Drawing for the job (mm, zero at the part's lowest x, y, z). A direction names the side the tool comes from. Give positions to 0.01 mm unless a question says otherwise; leave off trailing zeros. Write each loop counter-clockwise with the first axis right and the second up, starting at its lowest first coordinate (ties: lowest second). Pieces come first, ordered by that corner, then holes. Notation, with made-up numbers: M 1.25,-2.75 L 56.25,-2.75 A22 cw 56.25,24.25 Z; hole C 43.25,-3.5 d2. An arc over 180 degrees is marked long. Use CSV: the item, a comma, the result in double quotes. Start each with the question number.
1. Mould opens along X. For the marked faces 1, 2 and 3 say: pulls with the +X half, pulls with the -X half, needs draft (parallel to the pull), parting line crosses it, or undercut.
2. 3-axis set-ups, long thin cutter, end or side, ignore diameter. For the marked faces 4 and 5: which of +Z, -Z, +X, -X, +Y, -Y reach the whole face in a straight line?
3. Band-saw the part on A-A, the plane x = 12. List the corners of the cut face in (y, z).
4. Band-saw the part on C-C, the plane y = 0.5. List the corners of the cut face in (x, z), then the cut area to 3 significant figures.
5. Band-saw the part on D-D, the plane y = 8. List the corners of the cut face in (x, z).
6. Band-saw the part on B-B, the plane z = 12. List the corners of the cut face in (x, y), then the cut area to 3 significant figures.
7. Drop flat-ended pins along their axis: pin 1 Ø6 at (y, z) = (1, 17.5) entering from -X; pin 2 Ø8.5 at (x, z) = (12, 12) entering from -Y; pin 3 Ø1.5 at (y, z) = (9, 3) entering from -X. Give the stop position or say it passes through.
8. Drill centre lines: line 1 along Z through (x, y) = (12, 3.55); line 2 along Z through (x, y) = (12, 5.3). Where is each one in solid material? Low to high. Write a range as from..to.
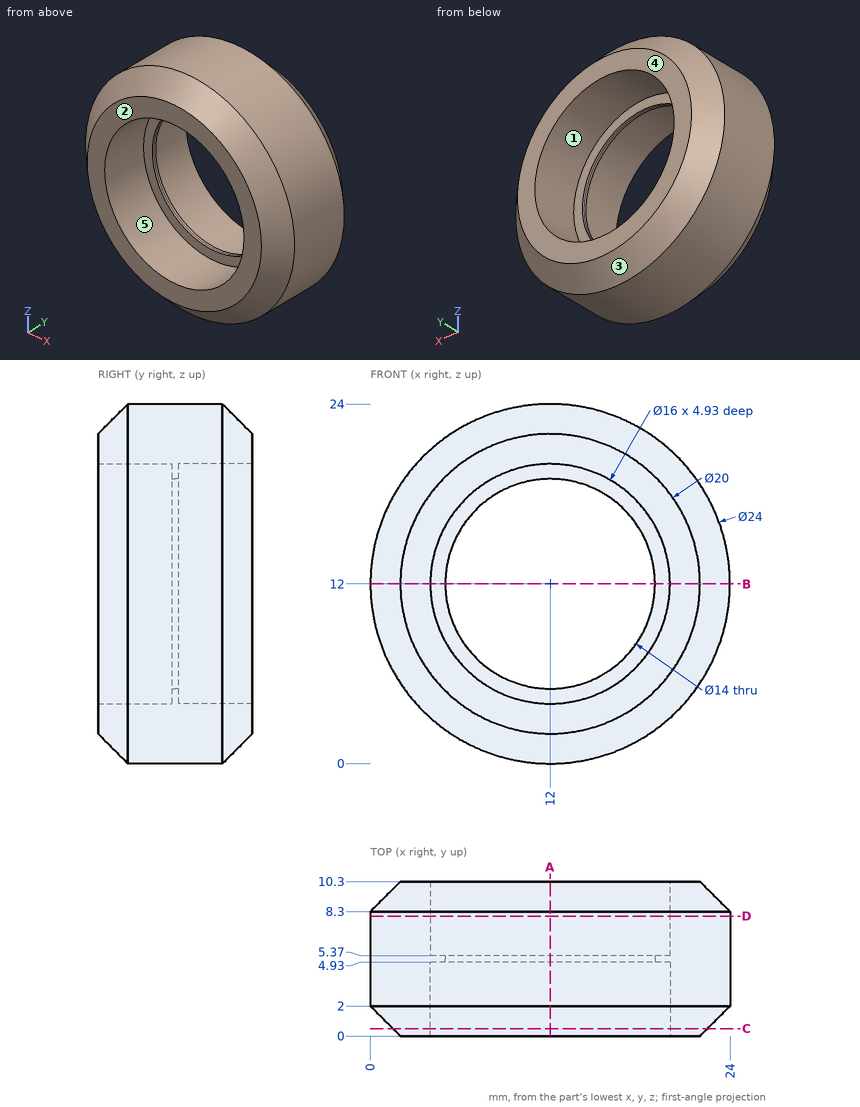
Output:
1,face 1,"undercut"
1,face 2,"needs draft"
1,face 3,"parting line crosses it"
2,face 4,"+Z, -Z, +X, -X, +Y"
2,face 5,"-Y"
3,outline,"M 0,2 L 2,0 L 8.3,0 L 10.3,2 L 10.3,4 L 5.37,4 L 5.37,5 L 4.93,5 L 4.93,4 L 0,4 Z; M 0,20 L 4.93,20 L 4.93,19 L 5.37,19 L 5.37,20 L 10.3,20 L 10.3,22 L 8.3,24 L 2,24 L 0,22 Z"
4,outline,"C 12,12 d21; hole C 12,12 d16"
4,area,"145 mm²"
5,outline,"C 12,12 d24; hole C 12,12 d16"
6,outline,"M 0,2 L 2,0 L 4,0 L 4,4.93 L 5,4.93 L 5,5.37 L 4,5.37 L 4,10.3 L 2,10.3 L 0,8.3 Z; M 19,4.93 L 20,4.93 L 20,0 L 22,0 L 24,2 L 24,8.3 L 22,10.3 L 20,10.3 L 20,5.37 L 19,5.37 Z"
6,area,"75.3 mm²"
7,pin 1,"stops at x = 0.3"
7,pin 2,"passes through"
7,pin 3,"stops at x = 3.72"
8,line 1,"z = 0..4, 20..24"
8,line 2,"z = 0..5, 19..24"
